Can you work these out from the model? Positions are in its coordinate system, mm. A direction names the side the tool comes from. Round coordinates to 2 decimals unless told otherwise and drop trailing zeros. Loops run counter-clockwise (first coordinate to the right, second up) from the corner with the lowest first, then second, coordinate; pieces in that order, holes last.
(1) I want a section at D-D on x = 12. Write out the boundary of the cut face in (y, z).
(2) I want a section at C-C on z = 15.25. Write out the boundary of the cut face in (x, y) (3 decimals).
(3) Thinking about a two-plate mould opening in Y: for faces 1 (the face through (-16, 0.5, 17)), 2 (the face through (-16, -0.5, 17)), 3 (the face through (-16, 0, 6)), 4 (the face through (0, 6.25, 11)), which applies, released by +Y, released by -Y, zero draft, split by the parting line, or undercut?
(4) If I drill on line 1 along Y through (x, z) = (15, 18); line 2 along Z through (x, y) = (-15.5, 1); line 3 along X through (y, z) = (0, 17.85) (3 decimals), over which ranges is the centre line in solid material (lowest first)?
(5) Which directions (+Z, -Z, +X, -X, +Y, -Y) give clear straight access to the entire face, cutting with the end or side of a thin tool? Please do faces 5 (the face through (7, 0, 22.5)), 6 (the face through (11.375, 0, 20)), 7 (the face through (0.908, -0.976, 26.996)), 8 (the face through (-16.375, 3, 17)).
(6) I want a section at B-B on y = -5.25. Write out the boundary of the cut face in (x, z) (3 decimals).
(7) Will these pins go through, and if not, where does the flat tip stop? pin 1 Ø5.5 at (x, y) = (-14, -2.5) entering from +Z; pin 2 Ø4 at (x, y) = (-15, 1) entering from -Z; pin 3 Ø12 at (x, z) = (1, 25) entering from +Y; pin 4 Ø1.2 at (y, z) = (-3.5, 17.5) entering from -X (3 decimals).
(8) I want a section at A-A on x = -10. Write out the boundary of the cut face in (y, z), plus the area to 3 significant figures.
from build123d import *

# Parameters (mm, degrees)
F0_W      = 22.75
F0_H      = 12.5
F1_DEPTH  = 22.5
F3_W      = 5
F3_H      = 12.5
F4_DEPTH  = 2.5
F6_DEPTH  = 2.5
F8_DEPTH  = 4.25
F9_R      = 1
F10_DEPTH = 1
F11_R     = 2.5
F12_DEPTH = 3
F14_DEPTH = 10
F15_R     = 0.5


with BuildPart() as f1:
    # F0 (on Top) → F1 (new body)
    with BuildSketch(Plane.XY):
        Rectangle(F0_W, F0_H)
    extrude(amount=F1_DEPTH)

    # F3 (on offset) → F4 (join)
    with BuildSketch(Plane.XY.offset(16)):
        with Locations((-13.875, 0)):
            Rectangle(F3_W, F3_H)
        with Locations((13.875, 0)):
            Rectangle(F3_W, F3_H)
    extrude(amount=F4_DEPTH)

    # F5 (on face) → F6 (cut, through all)
    with BuildSketch(Plane.XY.offset(18.5)):
        with BuildLine():
            Line((-16.375, -0.5), (-14.741025, -0.5))
            ThreePointArc((-14.741025, -0.5), (-12.875, 0), (-14.741025, 0.5))
            Line((-14.741025, 0.5), (-16.375, 0.5))
            Line((-16.375, 0.5), (-16.375, -0.5))
        make_face()
        with BuildLine():
            Line((16.375, 0.5), (14.741025, 0.5))
            ThreePointArc((14.741025, 0.5), (12.875, 0), (14.741025, -0.5))
            Line((14.741025, -0.5), (16.375, -0.5))
            Line((16.375, -0.5), (16.375, 0.5))
        make_face()
    extrude(amount=-F6_DEPTH, mode=Mode.SUBTRACT)

    # F7 (on face) → F8 (join)
    with BuildSketch(Plane.XY.offset(22.5)):
        with BuildLine():
            ThreePointArc((0.625, -2.44949), (3.625, 0), (0.625, 2.44949))
            ThreePointArc((0.625, 2.44949), (-1.678756, 5.21401), (-5.125, 6.25))
            ThreePointArc((-5.125, 6.25), (-9.544417, 4.419417), (-11.375, 0))
            ThreePointArc((-11.375, 0), (-9.544417, -4.419417), (-5.125, -6.25))
            ThreePointArc((-5.125, -6.25), (-1.678756, -5.21401), (0.625, -2.44949))
        make_face()
    extrude(amount=F8_DEPTH)

    # F9 (on face) → F10 (join)
    with BuildSketch(Plane.XY.offset(26.75)):
        with Locations((1.125, 0)):
            Circle(F9_R)
    extrude(amount=F10_DEPTH)

    # F11 (on face) → F12 (join)
    with BuildSketch(Plane.XY.offset(26.75)):
        with Locations((-5.125, 0)):
            Circle(F11_R)
    extrude(amount=F12_DEPTH)

    # F13 (on face) → F14 (join)
    with BuildSketch(Plane(origin=(-11.375, 0, 0), x_dir=(0, -1, 0), z_dir=(-1, 0, 0))):
        with BuildLine():
            Line((1.25, 6), (-1.25, 6))
            ThreePointArc((-1.25, 6), (-1.78033, 5.78033), (-2, 5.25))
            ThreePointArc((-2, 5.25), (-1.78033, 4.71967), (-1.25, 4.5))
            Line((-1.25, 4.5), (1.25, 4.5))
            ThreePointArc((1.25, 4.5), (1.78033, 4.71967), (2, 5.25))
            ThreePointArc((2, 5.25), (1.78033, 5.78033), (1.25, 6))
        make_face()
    extrude(amount=F14_DEPTH)

    # F15
    f15_edges = [f1.edges().sort_by_distance(p)[0] for p in [
        (0.125, 0, 27.75),
    ]]
    fillet(f15_edges, radius=F15_R)


solid = f1.part
Filled sheet:
1. outline: (-6.25, 16) - (6.25, 16) - (6.25, 18.5) - (-6.25, 18.5) - close
2. outline: (-11.375, -6.25) - (11.375, -6.25) - (11.375, 6.25) - (-11.375, 6.25) - close
3. face 1: undercut
3. face 2: undercut
3. face 3: zero draft
3. face 4: released by +Y
4. line 1: y = -6.25 to -0.5, 0.5 to 6.25
4. line 2: z = 4.5 to 6, 16 to 18.5
4. line 3: x = -12.875 to 12.875
5. face 5: +Z, +X
5. face 6: +Z, +X, +Y, -Y
5. face 7: +Z
5. face 8: +Z, -X, +Y, -Y
6. outline: (-16.375, 16) - (-11.375, 16) - (-11.375, 0) - (11.375, 0) - (11.375, 16) - (16.375, 16) - (16.375, 18.5) - (11.375, 18.5) - (11.375, 22.5) - (-1.734, 22.5) - (-1.734, 26.75) - (-8.516, 26.75) - (-8.516, 22.5) - (-11.375, 22.5) - (-11.375, 18.5) - (-16.375, 18.5) - close
7. pin 1: stops at z = 22.5
7. pin 2: stops at z = 4.5
7. pin 3: stops at y = 6.25
7. pin 4: stops at x = -16.375
8. outline: (-6.25, 0) - (6.25, 0) - (6.25, 22.5) - (3.91, 22.5) - (3.91, 26.75) - (-3.91, 26.75) - (-3.91, 22.5) - (-6.25, 22.5) - close
8. area: 314 mm2
